CAD build for the part. Positions are in the model's coordinates, mm. A direction names the side the tool comes from. Give positions to 0.01 mm unless a question says otherwise; leave off trailing zeros. Order: outer loops, then holes, each group sorted by start corner. A loop starts at its lowest first (then second) coordinate and runs counter-clockwise, first axis right, second up. Notation, with made-up numbers: (-37, -25.75) -> (6, -25.75) arc R12 cw to (6, -17.75) -> close; hole circle Ø11 at (8.5, -23.75). An arc over 180 degrees is marked (long way). Use one line per item in the form item = value. Start each with the question number.
1) Mould opens along Z. For faces 4 (the face through (47.869, 24, -16)), 5 (the face through (108, -10, 11.176)), 6 (the face through (90.45, -4.19, 0.11)) say: pulls with the +Z half, pulls with the -Z half, needs draft (parallel to the pull), parting line crosses it, or undercut.
2) Probe line 1 (Z direction, x = 110.5, y = -13); line 2 (Y direction, x = 69, z = 12); line 3 (Y direction, x = 38, z = 19.5). List the from-to ranges inside material, lowest first.
3) Tool access for faces 1 (the face through (60, 24, 4.318)), 2 (the face through (105, -14, 4.775)), 3 (the face through (39.233, 24, 16)): list every direction of +Z, -Z, +X, -X, +Y, -Y with a clear straight run to the whole face (end or side of a thin tool).
4) Cut at B-B, the plane x = 13.5. Give the cut face in (y, z).
5) Cut at A-A, the plane z = 2.5. State how many separate pieces and enclosed holes the cut face has, and give its area (3 significant figures).
6) Drop flat-ended pins along their axis: P1, Ø2.5, axis at x = 26.5, y = 23.5, coming from the -Z side; P2, Ø2, axis at y = 2, z = -14.5, coming from the +X side; P3, Ø1, axis at x = -15, z = -4, coming from the +Y side. Give the stop position or say it passes through.
from build123d import *

# Parameters (mm, degrees)
BOSS_EXTRUDE1_DEPTH                                  = 22.352
FILLET1_R                                            = 22.352
CUT_EXTRUDE1_DEPTH                                   = 136.349100872
BOSS_EXTRUDE2_START                                  = 6.35
BOSS_EXTRUDE2_DEPTH                                  = 6.35
SKETCH4_R                                            = 11.176
BOSS_EXTRUDE3_DEPTH                                  = 6.35
F_3_8_0_44_DIAMETER_HOLE1_D                          = 11.176
SKETCH7_R                                            = 20.701
BOSS_EXTRUDE4_DEPTH                                  = 16.002
CUT_EXTRUDE2_START                                   = -3.048
SKETCH8_W                                            = 8.636
SKETCH8_H                                            = 8.636
CUT_EXTRUDE2_DEPTH                                   = 3.048
CBORE_FOR_3_8_BINDING_HEAD_MACHINE_SCREW_D           = 10.414
CBORE_FOR_3_8_BINDING_HEAD_MACHINE_SCREW_CBORE_D     = 25.4
CBORE_FOR_3_8_BINDING_HEAD_MACHINE_SCREW_CBORE_DEPTH = 10.16
FILLET2_R                                            = 1.27


with BuildPart() as part:
    # Sketch1 → Boss-Extrude1 (new, symmetric)
    with BuildSketch(Plane.XY):
        Polygon((-23.756808877, -41.148), (0, 0), (70.477191123, 0), (128.643191123, -41.148), (134.217439977, -33.268351929), (73.546078299, 9.652), (-5.572584798, 9.652), (-32.115686074, -36.322), align=None)
    extrude(amount=BOSS_EXTRUDE1_DEPTH, both=True)

    # Fillet1
    fillet1_edges = [part.edges().sort_by_distance(p)[0] for p in [
        (-27.936247475, -38.735, 22.352),
        (-27.936247475, -38.735, -22.352),
        (131.43031555, -37.208175965, -22.352),
        (131.43031555, -37.208175965, 22.352),
    ]]
    fillet(fillet1_edges, radius=FILLET1_R - 0.0001)  # a hair under: the kernel refuses the full size

    # Sketch2 → Cut-Extrude1 (cut, through all)
    with BuildSketch(Plane(origin=(29.080678336, 41.107872463, 0), x_dir=(0.8163746447104718, -0.5775226744240014, 0), z_dir=(0.5775226744240014, 0.8163746447104718, 0))):
        with BuildLine():
            Line((106.432942455, -4.7752), (81.032942455, -4.7752))
            ThreePointArc((81.032942455, -4.7752), (76.257742455, 0), (81.032942455, 4.7752))
            Line((81.032942455, 4.7752), (106.432942455, 4.7752))
            ThreePointArc((106.432942455, 4.7752), (111.208142455, 0), (106.432942455, -4.7752))
        make_face()
    extrude(amount=-CUT_EXTRUDE1_DEPTH, mode=Mode.SUBTRACT)

    # Sketch3 → Boss-Extrude2 (add)
    with BuildSketch(Plane(origin=(29.080678336, 41.107872463, 0), x_dir=(0.8163746447104718, -0.5775226744240014, 0), z_dir=(0.5775226744240014, 0.8163746447104718, 0)).offset(BOSS_EXTRUDE2_START)):
        with BuildLine():
            Line((81.032942455, 11.176), (106.432942455, 11.176))
            ThreePointArc((106.432942455, 11.176), (117.608942455, 0), (106.432942455, -11.176))
            Line((106.432942455, -11.176), (81.032942455, -11.176))
            ThreePointArc((81.032942455, -11.176), (69.856942455, 0), (81.032942455, 11.176))
        make_face()
        with BuildLine():
            Line((81.032942455, 4.7752), (106.432942455, 4.7752))
            ThreePointArc((106.432942455, 4.7752), (111.208142455, 0), (106.432942455, -4.7752))
            Line((106.432942455, -4.7752), (81.032942455, -4.7752))
            ThreePointArc((81.032942455, -4.7752), (76.257742455, 0), (81.032942455, 4.7752))
        make_face(mode=Mode.SUBTRACT)
    extrude(amount=-BOSS_EXTRUDE2_DEPTH)

    # Sketch4 → Boss-Extrude3 (add)
    with BuildSketch(Plane(origin=(-8.358877197, 4.826, 0), x_dir=(0, 0, 1), z_dir=(-0.8660254037844402, 0.4999999999999977, 0))):
        with Locations(Location((0, -25.161617753, 0), (0, 0, 90))):
            Circle(SKETCH4_R)
    extrude(amount=BOSS_EXTRUDE3_DEPTH)

    # 3/8 (0.44) Diameter Hole1 (through all)
    with Locations(Plane(origin=(-13.858138511, 8.001, 0), x_dir=(0, 0, 1), z_dir=(-0.86602540378444, 0.49999999999999784, 0))):
        with Locations((0, -25.161617753)):
            Hole(F_3_8_0_44_DIAMETER_HOLE1_D / 2)

    # Sketch7 → Boss-Extrude4 (add)
    with BuildSketch(Plane(origin=(0, 9.652, 0), x_dir=(1, 0, 0), z_dir=(0, 1, 0))):
        with Locations(Location((43.551015202, 0, 0), (0, 0, 180))):
            Circle(SKETCH7_R)
    extrude(amount=BOSS_EXTRUDE4_DEPTH)

    # Sketch8 → Cut-Extrude2 (cut)
    with BuildSketch(Plane(origin=(0, 25.654, 0), x_dir=(1, 0, 0), z_dir=(0, 1, 0)).offset(CUT_EXTRUDE2_START)):
        with BuildLine():
            Line((39.233015202, 20.245648347), (39.233015202, 4.318))
            Line((39.233015202, 4.318), (47.869015202, 4.318))
            Line((47.869015202, 4.318), (47.869015202, 20.245648347))
            ThreePointArc((47.869015202, 20.245648347), (43.551015202, 20.701), (39.233015202, 20.245648347))
        make_face()
        with Locations((43.551015202, 0)):
            Rectangle(SKETCH8_W, SKETCH8_H)
        with BuildLine():
            Line((63.796663549, 4.318), (47.869015202, 4.318))
            Line((47.869015202, 4.318), (47.869015202, -4.318))
            Line((47.869015202, -4.318), (63.796663549, -4.318))
            ThreePointArc((63.796663549, -4.318), (64.137862549, -2.170971506), (64.252015202, 0))
            ThreePointArc((64.252015202, 0), (64.137862549, 2.170971506), (63.796663549, 4.318))
        make_face()
        with BuildLine():
            Line((47.869015202, -4.318), (39.233015202, -4.318))
            Line((39.233015202, -4.318), (39.233015202, -20.245648347))
            ThreePointArc((39.233015202, -20.245648347), (43.551015202, -20.701), (47.869015202, -20.245648347))
            Line((47.869015202, -20.245648347), (47.869015202, -4.318))
        make_face()
        with BuildLine():
            Line((39.233015202, 4.318), (23.305366855, 4.318))
            ThreePointArc((23.305366855, 4.318), (22.850015202, 0), (23.305366855, -4.318))
            Line((23.305366855, -4.318), (39.233015202, -4.318))
            Line((39.233015202, -4.318), (39.233015202, 4.318))
        make_face()
    extrude(amount=CUT_EXTRUDE2_DEPTH, mode=Mode.SUBTRACT)

    # CBORE for 3/8 Binding Head Machine Screw1 (through all)
    with Locations(Plane(origin=(0, 25.654, 0), x_dir=(1, 0, 0), z_dir=(0, 1, 0))):
        with Locations((43.551015202, 0)):
            CounterBoreHole(CBORE_FOR_3_8_BINDING_HEAD_MACHINE_SCREW_D / 2, CBORE_FOR_3_8_BINDING_HEAD_MACHINE_SCREW_CBORE_D / 2, CBORE_FOR_3_8_BINDING_HEAD_MACHINE_SCREW_CBORE_DEPTH)

    # Fillet2
    fillet2_edges = [part.edges().sort_by_distance(p)[0] for p in [
        (86.110114913, 0.763904229, 0),
        (105.601875931, -13.025027145, 11.176),
        (125.093636948, -26.81395852, 0),
        (105.601875931, -13.025027145, -11.176),
        (-26.527686074, -26.643300087, 0),
        (64.252015202, 9.652, 0),
    ]]
    fillet(fillet2_edges, radius=FILLET2_R)


solid = part.part
Result:
q1.face_4 = needs draft
q1.face_5 = pulls with the +Z half
q1.face_6 = undercut
q2.line_1 = -11.18 to -4.78, 4.78 to 11.18
q2.line_2 = 0 to 9.65
q2.line_3 = 0 to 25.65
q3.face_1 = +X, -X, +Y
q3.face_2 = none
q3.face_3 = +Z, -Z, +Y
q4.outline = (0, -22.35) -> (9.65, -22.35) -> (9.65, 22.35) -> (0, 22.35) -> close
q5.separate_pieces = 4
q5.enclosed_holes = 0
q5.area = 1,860 mm²
q6.P1 = -13.37
q6.P2 = 85.78
q6.P3 = -5.81
